from build123d import *

# Parameters (mm, degrees)
SKETCH1_W                = 84.708364016
SKETCH1_H                = 86.159780402
BOSS_EXTRUDE1_DEPTH      = 30
BOSS_EXTRUDE1_DEPTH_BACK = 30
FILLET1_R                = 30
FILLET2_R                = 20
FILLET3_R                = 10


with BuildPart() as part:
    # Sketch1 → Boss-Extrude1 (new body, two sides)
    with BuildSketch(Plane(origin=(0, 0, 0), x_dir=(1, 0, 0), z_dir=(0, 1, 0))) as boss_extrude1_sk:
        Rectangle(SKETCH1_W, SKETCH1_H)
    extrude(amount=BOSS_EXTRUDE1_DEPTH)
    extrude(boss_extrude1_sk.sketch, amount=-BOSS_EXTRUDE1_DEPTH_BACK)

    # Fillet1
    fillet1_edges = [part.edges().sort_by_distance(p)[0] for p in [
        (42.354182008, 0, 43.079890201),
        (-42.354182008, 0, 43.079890201),
        (-42.354182008, 0, -43.079890201),
        (42.354182008, 0, -43.079890201),
    ]]
    fillet(fillet1_edges, radius=FILLET1_R)

    # Fillet2
    fillet2_edges = [part.edges().sort_by_distance(p)[0] for p in [
        (0, 30, 43.079890201),
        (42.354182008, 30, 0),
        (0, 30, -43.079890201),
        (-42.354182008, 30, 0),
        (-33.567385444, 30, -34.293093637),
        (-33.567385444, 30, 34.293093637),
        (33.567385444, 30, -34.293093637),
        (33.567385444, 30, 34.293093637),
    ]]
    fillet(fillet2_edges, radius=FILLET2_R)

    # Fillet3
    fillet3_edges = [part.edges().sort_by_distance(p)[0] for p in [
        (0, -30, 43.079890201),
        (42.354182008, -30, 0),
        (-42.354182008, -30, 0),
        (0, -30, -43.079890201),
        (-33.567385444, -30, -34.293093637),
        (-33.567385444, -30, 34.293093637),
        (33.567385444, -30, -34.293093637),
        (33.567385444, -30, 34.293093637),
    ]]
    fillet(fillet3_edges, radius=FILLET3_R)


solid = part.part
Source: CAD feature listing. Evaluate the final solid. Frame: model axes, mm. Round coordinates to 2 decimals unless told otherwise and drop trailing zeros. Write each loop counter-clockwise with the first axis right and the second up, starting at its lowest first coordinate (ties: lowest second). Pieces come first, ordered by that corner, then holes. Notation, with made-up numbers: (-7.5, -3) - (15.5, -3) arc R22 cw to (15.5, 24) - close; hole circle Ø2 at (10, 9.5). An arc over 180 degrees is marked (long way). Use CSV: the item, a comma, the result in double quotes. Start each with the question number.
(1) Cut plane B-B, the plane x = -7. Return loops of the section in (y, z), and give its area (3 significant figures).
(2) First-contact query: pin 1 Ø3 at (x, y) = (-17, 3.5) entering from +Z; pin 2 Ø5 at (x, y) = (16, -9) entering from -Z; pin 3 Ø10 at (x, z) = (24.5, 29) entering from +Y. Flat tips, straight axial feed; report the tip coordinate or a pass-through.
(3) Cut plane A-A, the plane z = -4. Return loops of the section in (x, y), and give its area (3 significant figures).
(4) Material intervals for probe 1 along Y at (x, z) = (8, -24); probe 2 along X at (y, z) = (-13.5, -30); probe 3 along Z at (x, y) = (22, -14.5), sorted ascending. Write a range as [from, to].
Geometry says:
1,outline,"(-30, -33.08) arc R10 ccw to (-20, -43.08) - (10, -43.08) arc R20 ccw to (30, -23.08) - (30, 23.08) arc R20 ccw to (10, 43.08) - (-20, 43.08) arc R10 ccw to (-30, 33.08) - close"
1,area,"4,950 mm²"
2,pin 1,"z = 42.91"
2,pin 2,"z = -43.06"
2,pin 3,"y = 29.36"
3,outline,"(-42.35, -20) arc R10 ccw to (-32.35, -30) - (32.35, -30) arc R10 ccw to (42.35, -20) - (42.35, 10) arc R20 ccw to (22.35, 30) - (-22.35, 30) arc R20 ccw to (-42.35, 10) - close"
3,area,"4,870 mm²"
4,probe 1,"[-30, 29.98]"
4,probe 2,"[-37.13, 37.13]"
4,probe 3,"[-41.49, 41.49]"
